Design review of the part shown in the three views and the two pictorial views. Dimensions are in mm from the part's minimum x, y and z. Coordinates: 2 decimals unless noted, no trailing zeros. Write each loop counter-clockwise with the first axis right and the second up, starting at its lowest first coordinate (ties: lowest second). Pieces come first, ordered by that corner, then holes.
Q1. Take a section at C-C, the plane y = 1.7. Write out the cut boundary in (x, z), plus the area to 3 significant figures.
Q2. For pin 1 Ø1.5 at (y, z) = (1.5, 90.5) entering from -X, flat-tipped, find the tip position at first contact; note if it passes through.
Q3. For L1, parallel to Z at x = 29.5, y = 1.8; L2, parallel to X at y = 1.75, z = 108.5, list the stretches that pass through material, from the lowest coordinate up.
Q4. Take a section at B-B, the plane z = 47. Write out the cut boundary in (x, y).
Q5. Take a section at A-A, the plane x = 97. Write out the cut boundary in (y, z).
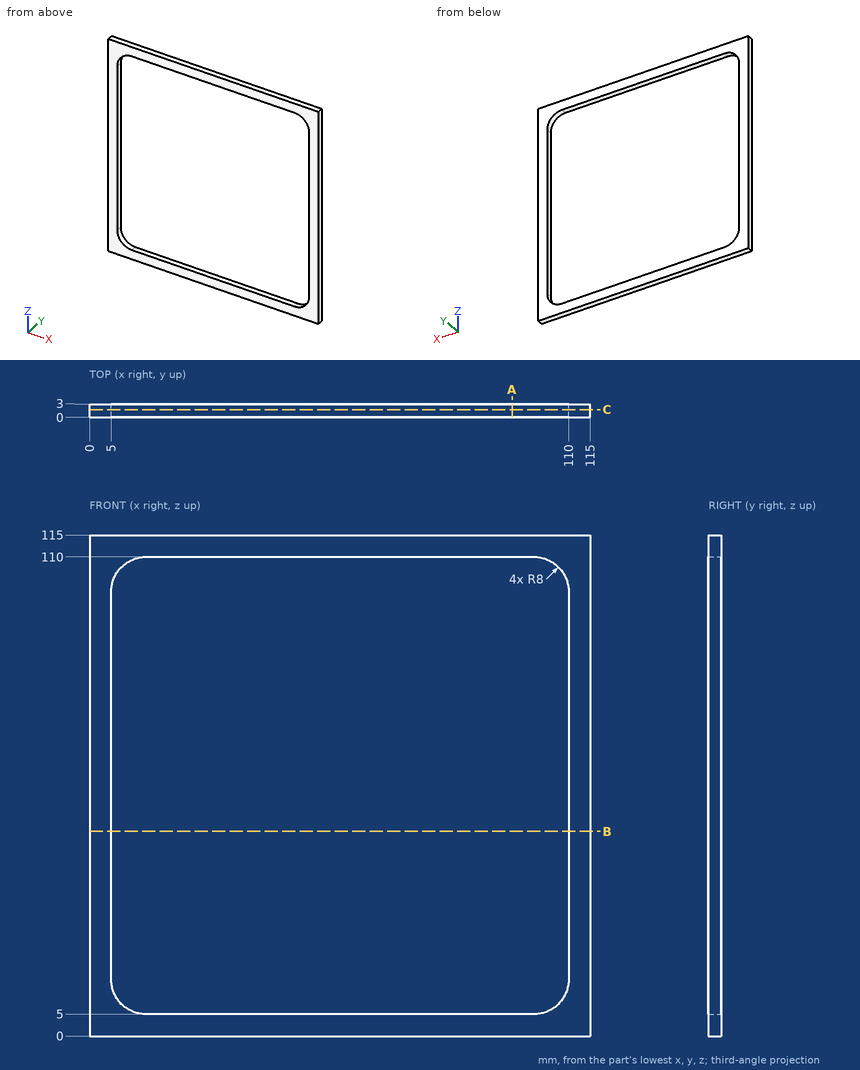
Responses:
1. outline: (0, 0) - (115, 0) - (115, 115) - (0, 115) - close; hole (5, 13) arc R8 ccw to (13, 5) - (102, 5) arc R8 ccw to (110, 13) - (110, 102) arc R8 ccw to (102, 110) - (13, 110) arc R8 ccw to (5, 102) - close
1. area: 2,250 mm2
2. pin 1: stops at x = 0
3. L1: z = 0 to 5, 110 to 115
3. L2: x = 0 to 8.34, 106.66 to 115
4. outline: (0, 0) - (5, 0) - (5, 3) - (0, 3) - close; (110, 0) - (115, 0) - (115, 3) - (110, 3) - close
5. outline: (0, 0) - (3, 0) - (3, 5) - (0, 5) - close; (0, 110) - (3, 110) - (3, 115) - (0, 115) - close
